from build123d import *

# Parameters (mm, degrees)
F0_R     = 15
F1_DEPTH = 150
F2_T     = -2.5
F3_R     = 5
F4_DEPTH = 25
F5_SIZE  = 2


with BuildPart() as f1:
    # F0 (on Top) → F1 (new body)
    with BuildSketch(Plane.XY):
        Circle(F0_R)
    extrude(amount=F1_DEPTH)

    # F2
    f2_openings = [f1.faces().sort_by_distance(p)[0] for p in [
        (0, 0, 150),
    ]]
    offset(amount=F2_T, openings=f2_openings)

    # F3 (on Top) → F4 (join)
    with BuildSketch(Plane.XY):
        Circle(F3_R)
    extrude(amount=-F4_DEPTH)

    # F5
    f5_edges = [f1.edges().sort_by_distance(p)[0] for p in [
        (-5, 0, -25),
    ]]
    chamfer(f5_edges, length=F5_SIZE)


solid = f1.part
Design review of the part built by this model. Coordinates are the model's own, in mm. A direction names the side the tool comes from. Round coordinates to 2 decimals unless told otherwise and drop trailing zeros. Loops run counter-clockwise (first coordinate to the right, second up) from the corner with the lowest first, then second, coordinate; pieces in that order, holes last. Notation, with made-up numbers: (-14.5, -16.75) -> (12.5, -16.75) arc R24 ccw to (12.5, 21.25) -> close; hole circle Ø4 at (39, 57). An arc over 180 degrees is marked (long way). Use one line per item in the form item = value. Start each with the question number.
Q1. We need section A-A on x = 0. Give the boundary of the cut face in (y, z), then the cut area to 3 significant figures.
Q2. We need section D-D on y = -8.5. Give the boundary of the cut face in (x, z), then the cut area to 3 significant figures.
Q3. Wall thickness on line 1 along Y through (x, z) = (0, 48.5); line 2 along X through (y, z) = (-0.5, 4); line 3 along Z through (x, y) = (10.25, -8.75): over which ranges is each line inside the solid? List them lowest first. Write a range as [from, to].
Q4. For pin 1 Ø10 at (y, z) = (6, 101.5) entering from -X; pin 2 Ø7.5 at (x, y) = (-1.5, -5) entering from +Z; pin 3 Ø6 at (y, z) = (-0.5, 36.5) entering from +X; pin 4 Ø1.5 at (x, y) = (5.5, -7) entering from -Z, all flat-tipped, find the tip position at first contact; note any pin that passes through.
Q5. Machinability: for faces 5 (the face through (-4, 4, 0)), 6 (the face through (-3.4, 12.3, 150)), which of the approach directions +Z, -Z, +X, -X, +Y, -Y give a long, thin tool a straight path to every point of the face, cutting with its end or side? Answer none if there is none.
Q6. Draft analysis for pull direction Y (two halves, no side actions). For faces 1 (the face through (0, 0, -25)), 2 (the face through (11.923, 3.755, 75.218)), 3 (the face through (0, 0, 2.5)), 4 (the face through (-1.08, -4.88, -11.34)), state which applies: +Y half, -Y half, draft (parallel to the pull), parting line (faces both ways), or undercut.
Q7. We need section C-C on z = 38.5. Give the boundary of the cut face in (x, y), then the cut area to 3 significant figures.
Calculated:
q1.outline = (-15, 0) -> (-5, 0) -> (-5, -23) -> (-3, -25) -> (3, -25) -> (5, -23) -> (5, 0) -> (15, 0) -> (15, 150) -> (12.5, 150) -> (12.5, 2.5) -> (-12.5, 2.5) -> (-12.5, 150) -> (-15, 150) -> close
q1.area = 1,060 mm²
q2.outline = (-12.36, 0) -> (12.36, 0) -> (12.36, 150) -> (9.17, 150) -> (9.17, 2.5) -> (-9.17, 2.5) -> (-9.17, 150) -> (-12.36, 150) -> close
q2.area = 1,000 mm²
q3.line_1 = [-15, -12.5], [12.5, 15]
q3.line_2 = [-14.99, -12.49], [12.49, 14.99]
q3.line_3 = [0, 150]
q4.pin_1 = -14.97
q4.pin_2 = 2.5
q4.pin_3 = 15
q4.pin_4 = 0
q5.face_5 = -Z
q5.face_6 = +Z, +X, -X, +Y, -Y
q6.face_1 = draft
q6.face_2 = undercut
q6.face_3 = undercut
q6.face_4 = parting line
q7.outline = circle Ø30 at (0, 0); hole circle Ø25 at (0, 0)
q7.area = 216 mm²
